Geometry check sheet. Reference: the model listing, model coordinates, mm. A direction names the side the tool comes from. Round coordinates to 2 decimals unless told otherwise and drop trailing zeros. Write each loop counter-clockwise with the first axis right and the second up, starting at its lowest first coordinate (ties: lowest second). Pieces come first, ordered by that corner, then holes. Notation, with made-up numbers: M 80.5,43.5 L 129.5,43.5 A9 cw 129.5,48.5 Z; hole C 39,24 d4. An arc over 180 degrees is marked long. One line per item, written item: value. Start each with the question number.
1. Access from +Z, -Z, +X, -X, +Y, -Y to the whole of each face (thin tool, end or side, straight path). Record for faces 1 (the cylindrical face through (-28.763, 4.216, -0.24)), 2 (the cylindrical face through (0, 11, 32)), 3 (the cylindrical face through (32, 11, 0)), 4 (the cylindrical face through (0, 7.5, -32.4)), 5 (the cylindrical face through (-32, 11, 0)).
2. Depth check by flat-ended pin: P1, Ø1.1, axis at y = 7.5, z = -31.5, coming from the +X side; P2, Ø2, axis at x = -1, y = 9, coming from the +Z side; P3, Ø1.5, axis at x = -6, z = -19, coming from the +Y side. Enter the tip coordinate at first touch or a pass-through.
3. Section check A-A (z = 0). Record the boundary of the cut face in (x, y).
4. Release check for a two-part mould opening along X. For faces 6 (the cylindrical face through (27.237, 4.216, -0.24)), 7 (the conical face through (28, 2, 0)), 8 (the cylindrical face through (0, 11, -32)), 9 (the flat face through (0.1, 13, 31.2)) record: pulls with the +X half, pulls with the -X half, needs draft (parallel to the pull), parting line crosses it, or undercut.
5. Scan lines: probe 1 along Z at (x, y) = (-0.5, 12.25); probe 2 along X at (y, z) = (9.5, -2.5); probe 3 along Y at (x, z) = (-15, -28). Record each from-to range of solid material in increasing order. Write a range as [from, to].
from build123d import *
from build123d.topology import SkipClean

# Parameters (mm, degrees)
SKETCH_1_R             = 35
EXTRUDE_1_DEPTH        = 6
EXTRUDE_1_TAPER        = 10
SKETCH_4_R             = 25
CUT_EXTRUDE_1_DEPTH    = 3
HOLE_WIZARD_M2_9_D     = 1.6
HOLE_WIZARD_M2_9_DEPTH = 3.519311505
HOLE_WIZARD_M2_9_TIP   = 0.480688495
SKETCH_21_R            = 33.942038116
EXTRUDE_2_DEPTH        = 4
EXTRUDE_2_TAPER        = 10
SKETCH_22_R            = 31
CUT_EXTRUDE_2_DEPTH    = 50.859803602
CUT_EXTRUDE_3_DEPTH    = 3
EXTRUDE_4_DEPTH        = 3


with BuildPart() as part:
    # Sketch 1 → Extrude 1 (new body)
    with BuildSketch(Plane(origin=(0, 0, 0), x_dir=(1, 0, 0), z_dir=(0, 1, 0))):
        Circle(SKETCH_1_R)
    extrude(amount=EXTRUDE_1_DEPTH, taper=EXTRUDE_1_TAPER)

    # Sketch 4 → Cut-Extrude 1 (cut)
    with BuildSketch(Plane(origin=(0, 6, 0), x_dir=(1, 0, 0), z_dir=(0, 1, 0))):
        with Locations(Location((0, 0, 0), (0, 0, 270))):
            Circle(SKETCH_4_R)
    extrude(amount=-CUT_EXTRUDE_1_DEPTH, mode=Mode.SUBTRACT)

    # Hole Wizard M2 _9
    with Locations(Plane(origin=(0, 6, 0), x_dir=(1, 0, 0), z_dir=(0, 1, 0))):
        with Locations((-28, 0), (28, 0)):
            Hole(HOLE_WIZARD_M2_9_D / 2, depth=HOLE_WIZARD_M2_9_DEPTH)
            with Locations((0, 0, -(HOLE_WIZARD_M2_9_DEPTH + HOLE_WIZARD_M2_9_TIP / 2))):  # 118° drill point
                Cone(0, HOLE_WIZARD_M2_9_D / 2, HOLE_WIZARD_M2_9_TIP, mode=Mode.SUBTRACT)

    # Sketch 21 → Extrude 2 (add)
    with BuildSketch(Plane(origin=(0, 6, 0), x_dir=(1, 0, 0), z_dir=(0, 1, 0))):
        Circle(SKETCH_21_R)
    extrude(amount=EXTRUDE_2_DEPTH, taper=EXTRUDE_2_TAPER)

    # Sketch 22 → Cut-Extrude 2 (cut, through all)
    with BuildSketch(Plane(origin=(0, 6, 0), x_dir=(1, 0, 0), z_dir=(0, 1, 0))):
        with Locations(Location((0, 0, 0), (0, 0, 270))):
            Circle(SKETCH_22_R)
    extrude(amount=CUT_EXTRUDE_2_DEPTH, mode=Mode.SUBTRACT)

    # Sketch 23 → Cut-Extrude 3 (cut)
    with BuildSketch(Plane(origin=(0, 6, 0), x_dir=(1, 0, 0), z_dir=(0, 1, 0))):
        with BuildLine():
            Line((-1.5, 32.365259152), (-1.5, 30.542622152))
            Line((-1.5, 30.542622152), (1.5, 30.542622152))
            Line((1.5, 30.542622152), (1.5, 32.365259152))
            ThreePointArc((1.5, 32.365259152), (0, 32.4), (-1.5, 32.365259152))
        make_face()
    extrude(amount=CUT_EXTRUDE_3_DEPTH, mode=Mode.SUBTRACT)

    # Sketch 31 → Extrude 4 (add)
    with SkipClean():  # the faces are left unmerged after this step: merging them gives an invalid solid
        with BuildSketch(Plane(origin=(0, 10, 0), x_dir=(1, 0, 0), z_dir=(0, 1, 0))):
            with BuildLine():
                Line((-8.282209443, 30.909626441), (-8.023390398, 29.943700615))
                ThreePointArc((-8.023390398, 29.943700615), (0, 31), (8.023390398, 29.943700615))
                Line((8.023390398, 29.943700615), (8.282209443, 30.909626441))
                ThreePointArc((8.282209443, 30.909626441), (0, 32), (-8.282209443, 30.909626441))
            make_face()
            with BuildLine():
                Line((30.909626441, -8.282209443), (29.943700615, -8.023390398))
                ThreePointArc((29.943700615, -8.023390398), (31, 0), (29.943700615, 8.023390398))
                Line((29.943700615, 8.023390398), (30.909626441, 8.282209443))
                ThreePointArc((30.909626441, 8.282209443), (32, 0), (30.909626441, -8.282209443))
            make_face()
            with BuildLine():
                Line((-8.282209443, -30.909626441), (-8.023390398, -29.943700615))
                ThreePointArc((-8.023390398, -29.943700615), (0, -31), (8.023390398, -29.943700615))
                Line((8.023390398, -29.943700615), (8.282209443, -30.909626441))
                ThreePointArc((8.282209443, -30.909626441), (0, -32), (-8.282209443, -30.909626441))
            make_face()
            with BuildLine():
                Line((-30.909626441, 8.282209443), (-29.943700615, 8.023390398))
                ThreePointArc((-29.943700615, 8.023390398), (-31, 0), (-29.943700615, -8.023390398))
                Line((-29.943700615, -8.023390398), (-30.909626441, -8.282209443))
                ThreePointArc((-30.909626441, -8.282209443), (-32, 0), (-30.909626441, 8.282209443))
            make_face()
        extrude(amount=EXTRUDE_4_DEPTH)


solid = part.part
Result sheet:
1. face 1: +Y
1. face 2: +Z, +Y
1. face 3: +X, +Y
1. face 4: none
1. face 5: -X, +Y
2. P1: stops at x = 13.3
2. P2: stops at z = 33.58
2. P3: stops at y = 3
3. outline: M -35,0 L 35,0 L 33.24,10 L 32,10 L 32,13 L 31,13 L 31,6 L 28.8,6 L 28.8,2.48 L 28,2 L 27.2,2.48 L 27.2,6 L 25,6 L 25,3 L -25,3 L -25,6 L -27.2,6 L -27.2,2.48 L -28,2 L -28.8,2.48 L -28.8,6 L -31,6 L -31,13 L -32,13 L -32,10 L -33.24,10 Z
4. face 6: undercut
4. face 7: undercut
4. face 8: parting line crosses it
4. face 9: needs draft
5. probe 1: z = [-32, -31], [31, 32]
5. probe 2: x = [-33.23, -30.9], [30.9, 33.23]
5. probe 3: y = [0, 10]
